Build history of the part. All positions in model axes, mm. Face numbers are marked on the shaded views. Round coordinates to 2 decimals unless told otherwise and drop trailing zeros. Order: outer loops, then holes, each group sorted by start corner. A loop starts at its lowest first (then second) coordinate and runs counter-clockwise, first axis right, second up. Notation, with made-up numbers: (55.25, -16) -> (113.25, -16) arc R19 cw to (113.25, 13) -> close; hole circle Ø2 at (-9.75, 47). An arc over 180 degrees is marked (long way). Answer as a JSON object with one key per item and string values.
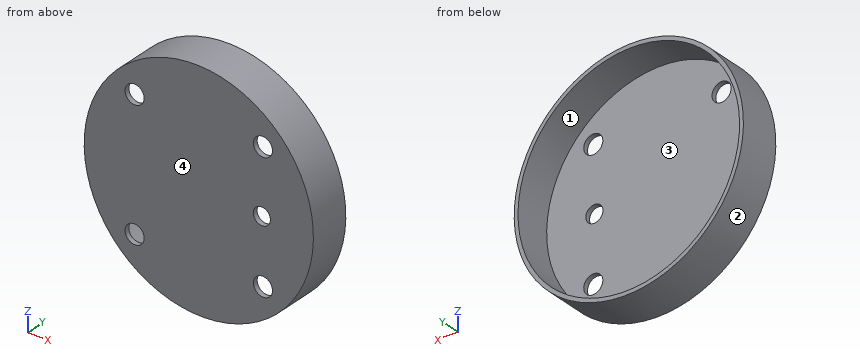
from build123d import *

# Parameters (mm, degrees)
SKETCH1_R           = 60
BOSS_EXTRUDE1_DEPTH = 2.5
SKETCH2_R           = 60
SKETCH2_R_2         = 58
BOSS_EXTRUDE2_DEPTH = 19
SKETCH3_R           = 4.5
SKETCH3_R_2         = 5
CUT_EXTRUDE1_DEPTH  = 87.954010833


with BuildPart() as part:
    # Sketch1 → Boss-Extrude1 (new body)
    with BuildSketch(Plane(origin=(0, 0, 0), x_dir=(1, 0, 0), z_dir=(0, 1, 0))):
        with Locations(Location((0, 0, 0), (0, 0, 270))):
            Circle(SKETCH1_R)
    extrude(amount=BOSS_EXTRUDE1_DEPTH)

    # Sketch2 → Boss-Extrude2 (add)
    with BuildSketch(Plane(origin=(0, 2.5, 0), x_dir=(1, 0, 0), z_dir=(0, 1, 0))):
        with Locations(Location((0, 0, 0), (0, 0, 270))):
            Circle(SKETCH2_R)
        with Locations(Location((0, 0, 0), (0, 0, 270))):
            Circle(SKETCH2_R_2, mode=Mode.SUBTRACT)
    extrude(amount=BOSS_EXTRUDE2_DEPTH)

    # Sketch3 → Cut-Extrude1 (cut, through all)
    with BuildSketch(Plane(origin=(0, 2.5, 0), x_dir=(1, 0, 0), z_dir=(0, 1, 0))):
        with Locations(Location((33, 0, 0), (0, 0, 270))):
            Circle(SKETCH3_R)
        with Locations(Location((33.587572106, 33.587572106, 0), (0, 0, 270))):
            Circle(SKETCH3_R_2)
        with Locations(Location((33.587572106, -33.587572106, 0), (0, 0, 270))):
            Circle(SKETCH3_R_2)
        with Locations(Location((-33.587572106, -33.587572106, 0), (0, 0, 270))):
            Circle(SKETCH3_R_2)
        with Locations(Location((-33.587572106, 33.587572106, 0), (0, 0, 270))):
            Circle(SKETCH3_R_2)
    extrude(amount=-CUT_EXTRUDE1_DEPTH, mode=Mode.SUBTRACT)


solid = part.part
1) Probe L1, parallel to Y at x = 54.5, z = 16; L2, parallel to Z at x = 50, y = 11; L3, parallel to X at y = 8.5, z = 17.5. List the from-to ranges inside material, lowest first. Write a range as from..to.
Checked values:
{"L1": "y = 0..2.5", "L2": "z = -33.17..-29.39, 29.39..33.17", "L3": "x = -57.39..-55.3, 55.3..57.39"}
2) Cut at C-C, the plane x = -37. Give the cut face in (y, z).
Checked values:
{"outline": "(0, -47.23) -> (21.5, -47.23) -> (21.5, -44.67) -> (2.5, -44.67) -> (2.5, -37.24) -> (0, -37.24) -> close; (0, -29.93) -> (2.5, -29.93) -> (2.5, 29.93) -> (0, 29.93) -> close; (0, 37.24) -> (2.5, 37.24) -> (2.5, 44.67) -> (21.5, 44.67) -> (21.5, 47.23) -> (0, 47.23) -> close"}
3) Cut at A-A, the plane x = 0. Give the cut face in (y, z), plus the area to 3 significant figures.
Checked values:
{"outline": "(0, -60) -> (21.5, -60) -> (21.5, -58) -> (2.5, -58) -> (2.5, 58) -> (21.5, 58) -> (21.5, 60) -> (0, 60) -> close", "area": "376 mm²"}
4) Pull direction Z, two halves, no side cores. Call the marked faces 1, 2, 3 and 4: pulls with the +Z half, pulls with the -Z half, needs draft (parallel to the pull), parting line crosses it, or undercut.
Checked values:
{"face 1": "undercut", "face 2": "parting line crosses it", "face 3": "undercut", "face 4": "needs draft"}
5) Cut at D-D, the plane y = 19. Give the cut face in (x, z), plus the area to 3 significant figures.
Checked values:
{"outline": "circle Ø120 at (0, 0); hole circle Ø116 at (0, 0)", "area": "741 mm²"}
6) Flat gauge pins, fed straight in: pin 1 Ø5 at (x, y) = (46, 3) entering from +Z; pin 2 Ø8 at (y, z) = (13.5, -31) entering from -X; pin 3 Ø2 at (x, y) = (-40.5, 11.5) entering from -Z. Where does each tip first touch, or does it go through?
Checked values:
{"pin 1": "stops at z = 41.32", "pin 2": "stops at x = -53.58", "pin 3": "stops at z = -45.16"}
7) Cut at B-B, the plane z = 0. Give the cut face in (x, y).
Checked values:
{"outline": "(-60, 0) -> (28.5, 0) -> (28.5, 2.5) -> (-58, 2.5) -> (-58, 21.5) -> (-60, 21.5) -> close; (37.5, 0) -> (60, 0) -> (60, 21.5) -> (58, 21.5) -> (58, 2.5) -> (37.5, 2.5) -> close"}
